```python
from build123d import *

# Parameters (mm, degrees)
CUT_EXTRUDE1_REACH = 4


with BuildPart() as part:
    # Sketch1 → Revolve1 (revolve)
    with BuildSketch(Plane.XY):
        with BuildLine():
            Line((-16.5, 9.4), (-18, 9.4))
            Line((-18, 9.4), (-18, 10.4))
            Line((-18, 10.4), (-16.5, 12))
            Line((-16.5, 12), (-16, 12))
            ThreePointArc((-16, 12), (-15.646446609, 11.853553391), (-15.5, 11.5))
            Line((-15.5, 11.5), (-15.5, 0))
            Line((-15.5, 0), (-10.75, 0))
            Line((-10.75, 0), (-10.75, -2))
            Line((-10.75, -2), (-18.5, -2))
            Line((-18.5, -2), (-18.5, 0))
            Line((-18.5, 0), (-18.5, 6))
            Line((-18.5, 6), (-19.5, 6))
            Line((-19.5, 6), (-19.5, 6.7))
            Line((-19.5, 6.7), (-17, 6.7))
            ThreePointArc((-17, 6.7), (-16.646446609, 6.846446609), (-16.5, 7.2))
            Line((-16.5, 7.2), (-16.5, 9.4))
        make_face()
    revolve(axis=Axis((0, 12.7, 0), (0, -1, 0)))

    # Sketch2 → Cut-Extrude1 (cut, up to next)
    with BuildSketch(Plane(origin=(0, 0, 0), x_dir=(1, 0, 0), z_dir=(0, 1, 0)), mode=Mode.PRIVATE) as cut_extrude1_sk1:
        with BuildLine():
            ThreePointArc((-13.984583698, 1.42392711), (-12.372295403, -6.672514973), (-6.49274382, -12.467575037))
            ThreePointArc((-6.49274382, -12.467575037), (-5.438109449, -12.135235565), (-5.770448921, -11.080601194))
            ThreePointArc((-5.770448921, -11.080601194), (-10.995921084, -5.930221166), (-12.42884798, 1.265520231))
            ThreePointArc((-12.42884798, 1.265520231), (-13.127512399, 2.12259153), (-13.984583698, 1.42392711))
        make_face()
    cut_extrude1_tool1 = extrude(cut_extrude1_sk1.sketch, amount=-CUT_EXTRUDE1_REACH, mode=Mode.PRIVATE) & part.part
    add(cut_extrude1_tool1.solids().sort_by_distance((-5.589512, 0, 12.05639))[0], mode=Mode.SUBTRACT)
    # Sketch2 → Cut-Extrude1 (cut, up to next)
    with BuildSketch(Plane(origin=(0, 0, 0), x_dir=(1, 0, 0), z_dir=(0, 1, 0)), mode=Mode.PRIVATE) as cut_extrude1_sk2:
        with BuildLine():
            ThreePointArc((1.42392711, 13.984583698), (-6.672514973, 12.372295403), (-12.467575037, 6.49274382))
            ThreePointArc((-12.467575037, 6.49274382), (-12.135235565, 5.438109449), (-11.080601194, 5.770448921))
            ThreePointArc((-11.080601194, 5.770448921), (-5.930221166, 10.995921084), (1.265520231, 12.42884798))
            ThreePointArc((1.265520231, 12.42884798), (2.12259153, 13.127512399), (1.42392711, 13.984583698))
        make_face()
    cut_extrude1_tool2 = extrude(cut_extrude1_sk2.sketch, amount=-CUT_EXTRUDE1_REACH, mode=Mode.PRIVATE) & part.part
    add(cut_extrude1_tool2.solids().sort_by_distance((-6.01125, 0, -11.146166))[0], mode=Mode.SUBTRACT)
    # Sketch2 → Cut-Extrude1 (cut, up to next)
    with BuildSketch(Plane(origin=(0, 0, 0), x_dir=(1, 0, 0), z_dir=(0, 1, 0)), mode=Mode.PRIVATE) as cut_extrude1_sk3:
        with BuildLine():
            ThreePointArc((13.984583698, -1.42392711), (12.372295403, 6.672514973), (6.49274382, 12.467575037))
            ThreePointArc((6.49274382, 12.467575037), (5.438109449, 12.135235565), (5.770448921, 11.080601194))
            ThreePointArc((5.770448921, 11.080601194), (10.995921084, 5.930221166), (12.42884798, -1.265520231))
            ThreePointArc((12.42884798, -1.265520231), (13.127512399, -2.12259153), (13.984583698, -1.42392711))
        make_face()
    cut_extrude1_tool3 = extrude(cut_extrude1_sk3.sketch, amount=-CUT_EXTRUDE1_REACH, mode=Mode.PRIVATE) & part.part
    add(cut_extrude1_tool3.solids().sort_by_distance((13.144804, 0, 1.952767))[0], mode=Mode.SUBTRACT)
    # Sketch2 → Cut-Extrude1 (cut, up to next)
    with BuildSketch(Plane(origin=(0, 0, 0), x_dir=(1, 0, 0), z_dir=(0, 1, 0)), mode=Mode.PRIVATE) as cut_extrude1_sk4:
        with BuildLine():
            ThreePointArc((-1.42392711, -13.984583698), (6.672514973, -12.372295403), (12.467575037, -6.49274382))
            ThreePointArc((12.467575037, -6.49274382), (12.135235565, -5.438109449), (11.080601194, -5.770448921))
            ThreePointArc((11.080601194, -5.770448921), (5.930221166, -10.995921084), (-1.265520231, -12.42884798))
            ThreePointArc((-1.265520231, -12.42884798), (-2.12259153, -13.127512399), (-1.42392711, -13.984583698))
        make_face()
    cut_extrude1_tool4 = extrude(cut_extrude1_sk4.sketch, amount=-CUT_EXTRUDE1_REACH, mode=Mode.PRIVATE) & part.part
    add(cut_extrude1_tool4.solids().sort_by_distance((6.01125, 0, 11.146166))[0], mode=Mode.SUBTRACT)


solid = part.part
```
CAD build for the part. Positions are in the model's coordinates, mm. A direction names the side the tool comes from. Round coordinates to 2 decimals unless told otherwise and drop trailing zeros. Order: outer loops, then holes, each group sorted by start corner. A loop starts at its lowest first (then second) coordinate and runs counter-clockwise, first axis right, second up. Notation, with made-up numbers: (22.5, 82) - (47.5, 82) arc R17 ccw to (47.5, 87) - close; hole circle Ø4 at (63.5, -15). An arc over 180 degrees is marked (long way). Use CSV: the item, a comma, the result in double quotes. Start each with the question number.
1) Pin check, flat tips, straight feed: pin 1 Ø8 at (x, y) = (-12.5, 6) entering from -Z; pin 2 Ø10 at (x, z) = (8, -0.5) entering from +Y; pin 3 Ø1.5 at (x, z) = (14, -15.5) entering from -Y; pin 4 Ø2 at (y, z) = (6.5, -15) entering from +X. Stop position of each tip, or through.
2) Tool access for faces 1 (the flat face through (-3.4, 0, -10.4)), 2 (the cylindrical face through (6.022, -0.986, 10.946)), 3 (the flat face through (16, 12, -3)): list every direction of +Z, -Z, +X, -X, +Y, -Y with a clear straight run to the whole face (end or side of a thin tool).
3) Two-plate mould, pull along X, no slides. Class faces 4 (the cylindrical face through (-10.946, -0.986, 6.022)), 5 (the flat face through (17.24, 6, 7.13)), 6 (the cylindrical face through (2.539, 6.355, -19.334)): pulls with the +X half, pulls with the -X half, needs draft (parallel to the pull), parting line crosses it, or undercut.
4) Saw through at B-B (y = 1.75). List the corners of the cut face in (x, z), and give its area (3 significant figures).
5) Saw through at A-A (x = 0). Count the separate pieces of the cut face and the enclosed holes in it, and give its area (3 significant figures).
6) Wall check: L1, parallel to X at y = -1.2, z = 0; L2, parallel to X at y = 2.75, z = 0. Give the ranges that are in metal, low to high. Write a range as [from, to].
Values follow:
1,pin 1,"stops at z = -17.55"
1,pin 2,"stops at y = 0"
1,pin 3,"passes through"
1,pin 4,"stops at x = 13.57"
2,face 1,"+Y"
2,face 2,"+Y, -Y"
2,face 3,"+Z, -Z, +X, -X, +Y"
3,face 4,"undercut"
3,face 5,"needs draft"
3,face 6,"parting line crosses it"
4,outline,"circle Ø37 at (0, 0); hole circle Ø31 at (0, 0)"
4,area,"320 mm2"
5,separate pieces,"4"
5,enclosed holes,"0"
5,area,"82.3 mm2"
6,L1,"x = [-18.5, -14.06], [-12.49, -10.75], [10.75, 12.49], [14.06, 18.5]"
6,L2,"x = [-18.5, -15.5], [15.5, 18.5]"
